```python
from build123d import *

# Parameters (mm, degrees)
F0_W     = 76.5
F0_H     = 28
F1_DEPTH = 3.6
F2_W     = 64.8
F2_H     = 16
F3_DEPTH = 25
F4_W     = 70.8
F4_H     = 23.3
F4_W_2   = 67.2
F4_H_2   = 19.8
F5_DEPTH = 2.8
F6_W     = 67.2
F6_H     = 19.8
F6_W_2   = 64.8
F6_H_2   = 16
F7_DEPTH = 1.6


with BuildPart() as f1:
    # F0 (on Top) → F1 (new body)
    with BuildSketch(Plane.XY):
        Rectangle(F0_W, F0_H)
    extrude(amount=F1_DEPTH)

    # F2 (on face) → F3 (cut)
    with BuildSketch(Plane.XY.offset(3.6)):
        Rectangle(F2_W, F2_H)
    extrude(amount=-F3_DEPTH, mode=Mode.SUBTRACT)

    # F4 (on face) → F5 (cut)
    with BuildSketch(Plane.XY.offset(3.6)):
        with Locations((0.4, 1.25)):
            Rectangle(F4_W, F4_H)
        with Locations((0.4, 1.3)):
            Rectangle(F4_W_2, F4_H_2, mode=Mode.SUBTRACT)
    extrude(amount=-F5_DEPTH, mode=Mode.SUBTRACT)

    # F6 (on face) → F7 (join)
    with BuildSketch(Plane.XY.offset(3.6)):
        with Locations((0.4, 1.3)):
            Rectangle(F6_W, F6_H)
        Rectangle(F6_W_2, F6_H_2, mode=Mode.SUBTRACT)
    extrude(amount=F7_DEPTH)


solid = f1.part
```
Geometry check sheet. Reference: the model listing, model coordinates, mm. A direction names the side the tool comes from. Give positions to 0.01 mm unless a question says otherwise; leave off trailing zeros. Write each loop counter-clockwise with the first axis right and the second up, starting at its lowest first coordinate (ties: lowest second). Pieces come first, ordered by that corner, then holes. Notation, with made-up numbers: (35.5, -9) -> (60.5, -9) arc R18 cw to (60.5, 0) -> close; hole circle Ø4 at (-11, 42.5). An arc over 180 degrees is marked (long way). Use one line per item in the form item = value.
Item 1: Depth check by flat-ended pin: pin 1 Ø2 at (x, z) = (-13.5, 4) entering from -Y. Enter the tip coordinate at first touch or a pass-through.
Results list:
pin_1 = -14
Item 2: Sectioned sample at C-C on y = 3.25. Enter the section's corners in (x, z), plus the area to 3 significant figures.
Results list:
outline = (-38.25, 0) -> (-32.4, 0) -> (-32.4, 5.2) -> (-33.2, 5.2) -> (-33.2, 0.8) -> (-35, 0.8) -> (-35, 3.6) -> (-38.25, 3.6) -> close; (32.4, 0) -> (38.25, 0) -> (38.25, 3.6) -> (35.8, 3.6) -> (35.8, 0.8) -> (34, 0.8) -> (34, 5.2) -> (32.4, 5.2) -> close
area = 35.9 mm2
Item 3: Sectioned sample at A-A on z = 2.6. Enter the section's corners in (x, y).
Results list:
outline = (-38.25, -14) -> (38.25, -14) -> (38.25, 14) -> (-38.25, 14) -> close; (-33.2, -8.6) -> (34, -8.6) -> (34, 11.2) -> (-33.2, 11.2) -> close; hole (-35, -10.4) -> (35.8, -10.4) -> (35.8, 12.9) -> (-35, 12.9) -> close; hole (-32.4, -8) -> (32.4, -8) -> (32.4, 8) -> (-32.4, 8) -> close
Item 4: Sectioned sample at B-B on x = -21. Enter the section's corners in (y, z).
Results list:
outline = (-14, 0) -> (-8, 0) -> (-8, 5.2) -> (-8.6, 5.2) -> (-8.6, 0.8) -> (-10.4, 0.8) -> (-10.4, 3.6) -> (-14, 3.6) -> close; (8, 0) -> (14, 0) -> (14, 3.6) -> (12.9, 3.6) -> (12.9, 0.8) -> (11.2, 0.8) -> (11.2, 5.2) -> (8, 5.2) -> close
Item 5: Access from +Z, -Z, +X, -X, +Y, -Y to the whole of each face (thin tool, end or side, straight path). Record for faces 4 (the flat face through (3, 9, 5.2)), 5 (the flat face through (-35, 1, 2)), 6 (the flat face through (32.4, 0, 3)).
Results list:
face_4 = +Z, +X, -X, +Y, -Y
face_5 = +Z
face_6 = +Z, -Z
Item 6: Scan lines: line 1 (Y direction, x = -18.5, z = 1.6); line 2 (X direction, y = -4.25, z = 2.15); line 3 (Y direction, x = -2, z = 4.2). Record each from-to range of solid material in increasing order.
Results list:
line_1 = -14 to -10.4, -8.6 to -8, 8 to 11.2, 12.9 to 14
line_2 = -38.25 to -35, -33.2 to -32.4, 32.4 to 34, 35.8 to 38.25
line_3 = -8.6 to -8, 8 to 11.2
Item 7: Mould release check, pull along Y, two halves, no side actions. Record for faces 1 (the flat face through (-1, 14, 2)), 2 (the flat face through (38.25, 0, 2)), 3 (the flat face through (0, -10.4, 2)): released by +Y, released by -Y, zero draft, split by the parting line, or undercut.
Results list:
face_1 = released by +Y
face_2 = zero draft
face_3 = undercut
